Could you check a few things on this model? Use its own coordinates, in mm. A direction names the side the tool comes from. Give positions to 0.01 mm unless a question says otherwise; leave off trailing zeros. Order: outer loops, then holes, each group sorted by start corner. A loop starts at its lowest first (then second) coordinate and runs counter-clockwise, first axis right, second up. Notation, with made-up numbers: M 66.25,16 L 92.25,16 A19 ccw 92.25,39 Z; hole C 50,39.5 d10. An arc over 180 degrees is marked long. Return JSON: item names as keys, results as strings. Group by question number.
Autodesk Inventor part; units mm, degrees
ref_plane "YZ Plane" through (0, 0, 0) normal (1, 0, 0) x (0, 1, 0)
ref_plane "XZ Plane" through (0, 0, 0) normal (0, 1, 0) x (-1, 0, 0)
ref_plane "XY Plane" through (0, 0, 0) normal (0, 0, 1) x (1, 0, 0)
sketch "Skizze1" plane through (0, 0, 0) normal (1, 0, 0) x (0, 1, 0)
  line L0 (-10, -10) -> (-10, -5)
  line L1 (-10, -5) -> (-15, -5)
  line L2 (-15, -5) -> (-15, 0)
  line L3 (-15, 0) -> (15, 0)
  line L4 (15, 0) -> (15, -5)
  line L5 (15, -5) -> (10, -5)
  line L6 (10, -5) -> (10, -10)
  line L7 (10, -10) -> (20, -10)
  line L8 (20, -10) -> (20, -30)
  line L9 (20, -30) -> (-20, -30)
  line L10 (-20, -30) -> (-20, -10)
  line L11 (-20, -10) -> (-10, -10)
  line L12 (0, -36) -> (0, 6)
  point P0 (0, 0)
  dimension "d0" = 30
  dimension "d1" = 20
  dimension "d2" = 5
  dimension "d3" = 5
  dimension "d4" = 20
  dimension "d5" = 90
  dimension "d6" = 40
extrude "Extrusion1" add sketch "Skizze1" along normal blind 10
sketch "Skizze3" plane through (0, 20, -10) normal (0, 1, 0) x (1, 0, 0)
  line L0 (0, 0) -> (0, 20)
  line L1 (0, 20) -> (40, 20)
  line L2 (40, 20) -> (40, 80)
  line L3 (40, 80) -> (-10, 80)
  line L4 (-10, 80) -> (-10, 90)
  line L5 (-10, 90) -> (50, 90)
  line L6 (50, 90) -> (50, 10)
  line L7 (50, 10) -> (0, 10)
  point P0 (0, -10)
  dimension "d12" = 10
  dimension "d13" = 10
  dimension "d14" = 10
  dimension "d15" = 60
  dimension "d16" = 50
  dimension "d17" = 60
extrude "Extrusion3" add sketch "Skizze3" against normal up to surface (40 mm away)
sketch "Skizze4" plane through (50, 20, -100) normal (0, 0, -1) x (-1, 0, 0)
  arc A0 (53.3975, 30) -> (53.3975, -70) centre (140, -20) ccw
  arc A1 (62.0577, 25) -> (62.0577, -65) centre (140, -20) ccw
  line L0 (140, -20) -> (53.3975, -70)
  line L1 (140, -20) -> (53.3975, 30)
  line L2 (0, -40) -> (60, -40)
  line L3 (0, 0) -> (60, 0)
  line L4 (0, 0) -> (0, -40)
  point P0 (40, -20)
  point P1 (42.0204, 0)
  point P2 (52.2504, 0)
  point P3 (52.2504, -40)
  point P4 (42.0204, -40)
  dimension "d20" = 200
  dimension "d21" = 180
  dimension "d22" = 30
  dimension "d23" = 30
  dimension "d24" = 40
  dimension "d25" = 20
  dimension "d30" = 140
extrude "Extrusion4" add sketch "Skizze4" against normal up to surface (10 mm away) contours L1 A1 L3 A0 | L2 A1 L0 A0
sketch "Skizze5" plane through (40, -20, -90) normal (0, 0, 1) x (1, 0, 0)
  arc A0 (-42.2504, 40) -> (-52.0577, 65) centre (-130, 20) ccw
  circle A1 centre (-130, 20) radius 90
  point P0 (-40, 20)
  point P1 (-52.0577, 65)
  point P2 (-42.2504, 40)
extrude "Extrusion5" cut sketch "Skizze5" against normal up to surface (10 mm away)
sketch "Skizze6" plane through (40, -20, -90) normal (0, 0, 1) x (1, 0, 0)
  line L0 (-30, 0) -> (-30, 40)
  line L1 (-30, 0) -> (10, 0)
  line L2 (10, 40) -> (10, 0)
  line L3 (-30, 40) -> (10, 40)
  arc A0 (-52.0577, -25) -> (-52.0577, 65) centre (-130, 20) ccw
  line L4 (-43.3975, -30) -> (-52.0577, -25)
  arc A1 (-43.3975, -30) -> (-32.0204, 0) centre (-130, 20) ccw
  line L5 (-32.0204, 0) -> (0, 0)
  line L6 (0, 40) -> (0, 0)
  line L7 (-32.0204, 40) -> (0, 40)
  arc A2 (-32.0204, 40) -> (-43.3975, 70) centre (-130, 20) ccw
  line L8 (-52.0577, 65) -> (-43.3975, 70)
  point P0 (-40, 20)
  point P1 (-30, 0)
  point P2 (-30, 40)
extrude "Extrusion6" cut sketch "Skizze6" against normal through all
equation "\"d13\" = d12"
equation "\"d23\" = d22"
equation "\"d25\" = 0.5 * d24"
properties part number "Finger"
1. Imagine slicing it at D-D, the plane y = 16. Please give me the cut outline in (x, z).
2. For pin 1 (12 mm diameter, centred on x = 9, y = 5, fed in from -Z); pin 2 (20 mm diameter, centred on x = 23.5, y = -6.5, fed in from +Z); pin 3 (2.5 mm diameter, centred on x = 3.5, z = -1.5, fed in from +Y), each with a flat end and sliding along its axis, tell me the tip position at first contact or that it passes through.
3. Which directions (+Z, -Z, +X, -X, +Y, -Y) give clear straight access to the entire face, cutting with the end or side of a thin tool? Please do faces 4 (the flat face through (30, 0, -20)), 5 (the flat face through (5, 10, -7)), 6 (the flat face through (5, -15, -10)), 7 (the flat face through (40, 0, -60)).
4. Imagine slicing it at C-C, the plane z = -33.5. Please give me the cut outline in (x, y), plus the area to 3 significant figures.
5. If we mould it in two halves opening along Z, with no side actions, what happens to faces 1 (the flat face through (5, 15, -2)), 2 (the flat face through (5, -10, -8)), 3 (the flat face through (20, 0, -30))? For each: pulls with the +Z half, pulls with the -Z half, needs draft (parallel to the pull), parting line crosses it, or undercut.
6. Imagine slicing it at A-A, the plane y = -5. Please give me the cut outline in (x, z).
7. Imagine slicing it at B-B, the plane x = 8.5. Please give me the cut outline in (y, z).
8. I need wall thicknesses on L1, parallel to Z at x = 3.5, y = 13; L2, parallel to X at y = 0.5, z = -17.5; L3, parallel to Z at x = 34.5, y = 8.5. Which ranges of each line are inside material? Lowest first, please. Write a range as from..to.
Values:
{
 "1": {"outline": "M 0,-30 L 40,-30 L 40,-90 L 50,-90 L 50,-20 L 10,-20 L 10,-10 L 0,-10 Z"},
 "2": {"pin 1": "stops at z = -30", "pin 2": "stops at z = -20", "pin 3": "stops at y = 15"},
 "3": {"face 4": "+Z, +X, +Y, -Y", "face 5": "+X, -X, +Y", "face 6": "+X, -X, -Y", "face 7": "-Z, -X, +Y, -Y"},
 "4": {"outline": "M 40,-20 L 50,-20 L 50,20 L 40,20 Z", "area": "400 mm²"},
 "5": {"face 1": "needs draft", "face 2": "undercut", "face 3": "pulls with the -Z half"},
 "6": {"outline": "M 0,-30 L 40,-30 L 40,-90 L 50,-90 L 50,-20 L 10,-20 L 10,0 L 0,0 Z"},
 "7": {"outline": "M -20,-30 L 20,-30 L 20,-10 L 10,-10 L 10,-5 L 15,-5 L 15,0 L -15,0 L -15,-5 L -10,-5 L -10,-10 L -20,-10 Z"},
 "8": {"L1": "z = -30..-10, -5..0", "L2": "x = 0..10", "L3": "z = -30..-20"}
}
